For this review, take the finished solid that the model builds, in its own axes (mm). Round coordinates to 2 decimals unless told otherwise and drop trailing zeros. Write each loop counter-clockwise with the first axis right and the second up, starting at its lowest first coordinate (ties: lowest second). Pieces come first, ordered by that corner, then holes. Notation, with made-up numbers: M 4.25,-37 L 34.25,-37 A9 ccw 34.25,-24 Z; hole C 81.5,59.5 d9. An arc over 180 degrees is marked long. Answer in a Markdown table with one row per item.
Autodesk Inventor part; units mm, degrees
ref_plane "YZ Plane" through (0, 0, 0) normal (1, 0, 0) x (0, 1, 0)
ref_plane "XZ Plane" through (0, 0, 0) normal (0, 1, 0) x (-1, 0, 0)
ref_plane "XY Plane" through (0, 0, 0) normal (0, 0, 1) x (1, 0, 0)
sketch "Эскиз1" plane through (0, 0, 0) normal (1, 0, 0) x (0, 1, 0)
  circle A0 centre (0, 0) radius 4
  circle A1 centre (0, 0) radius 1.5
  dimension "d0" = 8
  dimension "d1" = 3
extrude "Выдавливание1" add sketch "Эскиз1" along normal mid plane 308 contours A0 | A1
sketch "Эскиз2" plane through (154, 0, 0) normal (1, 0, 0) x (0, 0, -1)
  circle A0 centre (0, 0) radius 1.5
  dimension "d4" = 3
extrude "Выдавливание2" cut sketch "Эскиз2" against normal blind 8
sketch "Эскиз3" plane through (-154, 0, 0) normal (-1, 0, 0) x (0, 0, 1)
  circle A0 centre (0, 0) radius 1.5
  dimension "d7" = 3
extrude "Выдавливание3" cut sketch "Эскиз3" against normal blind 8
chamfer "Фаска1" distance 0.5 angle 45 2 edges at (-154, -4, 0) (154, -4, 0)
properties part number "вал 8мм ось x"
Q1. Mouldability with a two-part tool opening along Y and no side actions: class faces 1 (the face through (2.149, -0.867, -3.905)), 2 (the face through (-154, 0, -2)) as +Y half, -Y half, draft (parallel to the pull), parting line (faces both ways), or undercut.
Found:
| item | result |
|---|---|
| face 1 | parting line |
| face 2 | draft |
Q2. For probe 1 along Z at (x, y) = (-45, 0.25); probe 2 along Y at (x, z) = (32, -0.5); probe 3 along X at (y, z) = (0, 0), list the stretches that pass through material, from the lowest coordinate up.
Found:
| item | result |
|---|---|
| probe 1 | -3.99 to 3.99 |
| probe 2 | -3.97 to 3.97 |
| probe 3 | -146 to 146 |
Q3. Take a section at A-A (z = 0). State the section outline as (x, y) points, then the cut area to 3 significant figures.
Found:
| item | result |
|---|---|
| outline | M -154,-3.5 L -153.5,-4 L 153.5,-4 L 154,-3.5 L 154,-1.5 L 146,-1.5 L 146,1.5 L 154,1.5 L 154,3.5 L 153.5,4 L -153.5,4 L -154,3.5 L -154,1.5 L -146,1.5 L -146,-1.5 L -154,-1.5 Z |
| area | 2,420 mm² |
Q4. Take a section at C-C (x = -48). State the section outline as (y, z) points, then the cut area to 3 significant figures.
Found:
| item | result |
|---|---|
| outline | C 0,0 d8 |
| area | 50.3 mm² |
Q5. Insertion check: P1, Ø3.5, axis at y = 0, z = 0, coming from the -X side; P2, Ø3, axis at x = 52, z = 2.5, coming from the -Y side; P3, Ø1.5, axis at y = 0, z = 0.5, coming from the -X side; P4, Ø2, axis at x = -13, y = 2.5, coming from the -Z side. Each pin has a flat end and moves straight along its axis. Give the tip position at first contact, or say it passes through.
Found:
| item | result |
|---|---|
| P1 | x = -154 |
| P2 | y = -3.87 |
| P3 | x = -146 |
| P4 | z = -3.71 |
